Part print with two shaded views. Sizes in mm from the minimum x, y, z corner. A direction names the side the tool comes from. Round coordinates to 2 decimals unless told otherwise and drop trailing zeros. Loops run counter-clockwise (first coordinate to the right, second up) from the corner with the lowest first, then second, coordinate; pieces in that order, holes last. Notation, with made-up numbers: M -26.5,15.25 L -11.5,15.25 A25 ccw -11.5,36.25 Z; hole C 5.5,-29 d3. An arc over 180 degrees is marked long. Answer as CSV lines item,"result". Start each with the question number.
Item 1: Wall check: line 1 (Y direction, x = 16, z = 0.7); line 2 (Y direction, x = 11, z = 0.95); line 3 (X direction, y = 16.25, z = 3.4). Give the ranges that are in metal, low to high.
Item 2: Band-saw the part on C-C (y = 17). Give the cut face in (x, z), and give its area (3 significant figures).
Item 3: Band-saw the part on A-A (z = 4.6). Give the cut face in (x, y).
Item 4: Drop flat-ended pins along their axis: pin 1 Ø1.5 at (y, z) = (17.5, 3.5) entering from +X; pin 2 Ø1.5 at (y, z) = (19, 1.5) entering from -X; pin 3 Ø2.5 at (y, z) = (7.5, 3) entering from -X. Give the stop position or say it passes through.
Item 5: Which spindle directions (+Z, -Z, +X, -X, +Y, -Y) get a long thin tool onto all of the face, cutting with end or side? Do the marked faces 1 and 2. Say none if no direction does.
Item 6: Band-saw the part on D-D (x = 5). Give the cut face in (y, z).
Item 7: Band-saw the part on B-B (x = 12.5). Give the cut face in (y, z).
Item 8: Mould opens along X. For the marked faces 3, 4, 5 and 6 say: pulls with the +X half, pulls with the -X half, needs draft (parallel to the pull), parting line crosses it, or undercut.
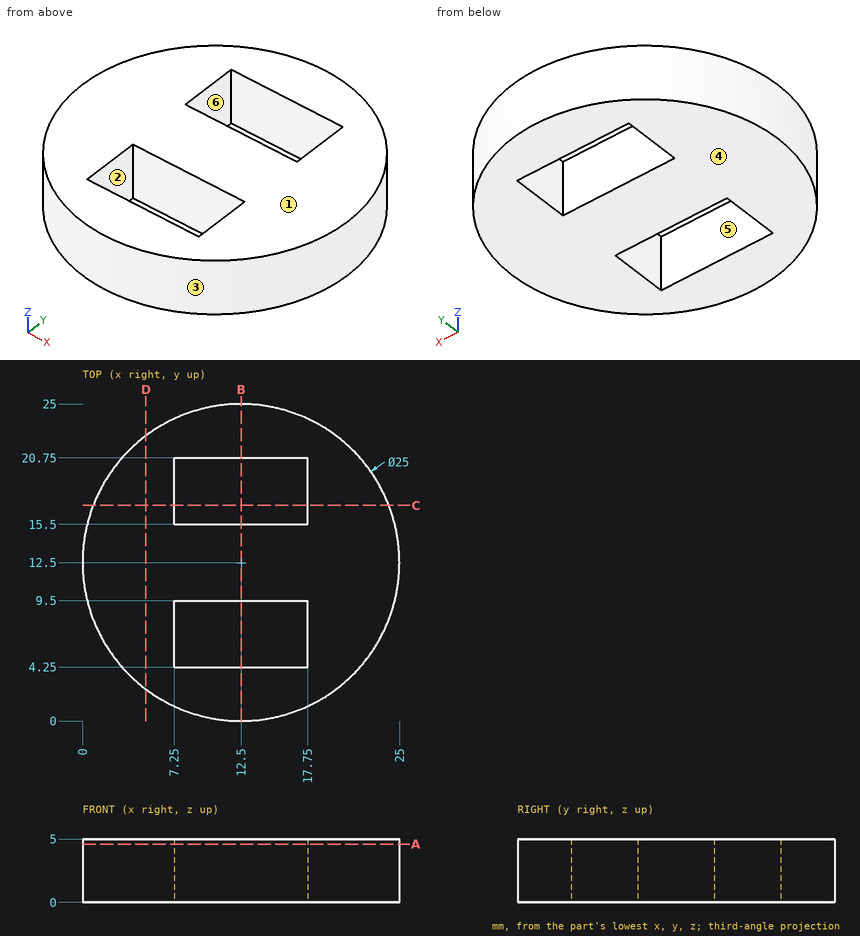
Answer block:
1,line 1,"y = 0.5 to 4.25, 9.5 to 15.5, 20.75 to 24.5"
1,line 2,"y = 0.09 to 4.25, 9.5 to 15.5, 20.75 to 24.91"
1,line 3,"x = 0.58 to 7.25, 17.75 to 24.42"
2,outline,"M 0.84,0 L 7.25,0 L 7.25,5 L 0.84,5 Z; M 17.75,0 L 24.16,0 L 24.16,5 L 17.75,5 Z"
2,area,"64.1 mm^2"
3,outline,"C 12.5,12.5 d25; hole M 7.25,4.25 L 17.75,4.25 L 17.75,9.5 L 7.25,9.5 Z; hole M 7.25,15.5 L 17.75,15.5 L 17.75,20.75 L 7.25,20.75 Z"
4,pin 1,"stops at x = 24.26"
4,pin 2,"stops at x = 1.4"
4,pin 3,"stops at x = 0.58"
5,face 1,"+Z, +X, -X, +Y, -Y"
5,face 2,"+Z, -Z"
6,outline,"M 2.5,0 L 22.5,0 L 22.5,5 L 2.5,5 Z"
7,outline,"M 0,0 L 4.25,0 L 4.25,5 L 0,5 Z; M 9.5,0 L 15.5,0 L 15.5,5 L 9.5,5 Z; M 20.75,0 L 25,0 L 25,5 L 20.75,5 Z"
8,face 3,"parting line crosses it"
8,face 4,"needs draft"
8,face 5,"undercut"
8,face 6,"undercut"
